Autodesk Inventor part; units mm, degrees
ref_plane "YZ Plane" through (0, 0, 0) normal (1, 0, 0) x (0, 1, 0)
ref_plane "XZ Plane" through (0, 0, 0) normal (0, 1, 0) x (-1, 0, 0)
ref_plane "XY Plane" through (0, 0, 0) normal (0, 0, 1) x (1, 0, 0)
sketch "Sketch1" plane through (0, 0, 0) normal (0, 1, 0) x (-1, 0, 0)
  circle A0 centre (0, 0) radius 40
  dimension "d0" = 80
extrude "Extrusion1" add sketch "Sketch1" along normal blind 6
sketch "Sketch2" plane through (0, 0, 0) normal (0, -1, 0) x (1, 0, 0)
  circle A0 centre (0, 0) radius 35.15
  circle A1 centre (0, 0) radius 24.85
  point P0 (0, 0)
extrude "Extrusion2" cut sketch "Sketch2" against normal blind 1.43
sketch "Sketch3" plane through (0, 6, 0) normal (0, 1, 0) x (1, 0, 0)
  circle A0 centre (-7, 0) radius 0.7835
  circle A1 centre (0, 7) radius 0.7835
  circle A2 centre (0, -7) radius 0.7835
  circle A3 centre (7, 0) radius 0.7835
  point P0 (0, 0)
hole "Hole1" at (-7, 6, 0) at (0, 6, 7) at (7, 6, 0) at (0, 6, -7) direction (0, -1, 0) diameter 2.1 end through all
sketch "Sketch4" plane through (0, 6, 0) normal (0, 1, 0) x (1, 0, 0)
  circle A0 centre (0, 7) radius 1.05
  circle A1 centre (7, 0) radius 1.05
  circle A2 centre (0, -7) radius 1.05
  circle A3 centre (-7, 0) radius 1.05
  circle A4 centre (0, 0) radius 40
  circle A5 centre (-7, 0) radius 2.05
  circle A6 centre (0, -7) radius 2.05
  circle A7 centre (7, 0) radius 2.05
  circle A8 centre (0, 7) radius 2.05
  dimension "d12" = 4.1
extrude "Extrusion3" cut sketch "Sketch4" against normal blind 3 contours A5 | A6 | A7 | A8
sketch "Sketch5" plane through (0, 6, 0) normal (0, 1, 0) x (1, 0, 0)
  circle A0 centre (0, 0) radius 1.75
  circle A1 centre (0, 0) radius 2
  dimension "d27" = 4
extrude "Extrusion4" cut sketch "Sketch5" against normal through all contours A0 | A1
sketch "Sketch6" plane through (0, 0, 0) normal (0, -1, 0) x (1, 0, 0)
  circle A0 centre (0, 0) radius 3
  dimension "d17" = 6
extrude "Extrusion5" cut sketch "Sketch6" against normal blind 1.5
sketch "Sketch7" plane through (0, 6, 0) normal (0, 1, 0) x (1, 0, 0)
  circle A0 centre (-4, -36.56) radius 1.05
  circle A1 centre (-4, -27.06) radius 1.05
  circle A2 centre (14, -27.06) radius 1.05
  circle A3 centre (14, -34.56) radius 1.05
  circle A4 centre (18, 25.06) radius 1.05
  circle A5 centre (18, 32.06) radius 1.05
  circle A6 centre (0, 35.06) radius 1.05
  circle A7 centre (0, 25.06) radius 1.05
  circle A8 centre (-18, 32.06) radius 1.05
  circle A9 centre (-18, 25.06) radius 1.05
  point P0 (0, 0)
hole "Hole2" at (-18, 6, -32.06) at (0, 6, -35.06) at (18, 6, -32.06) at (18, 6, -25.06) at (0, 6, -25.06) at (-18, 6, -25.06) at (-4, 6, 27.06) at (14, 6, 27.06) at (14, 6, 34.56) at (-4, 6, 36.56) direction (0, -1, 0) diameter 1.567 depth 3
properties part number "axis_2_bottom_frame" material "Aluminum 6061-AHC"
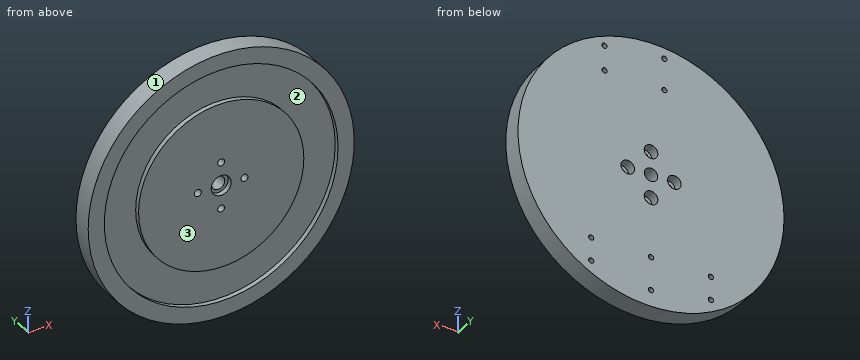
Design review of the part built by this model. Coordinates are the model's own, in mm. Face numbers are marked on the shaded views. Coordinates: 2 decimals unless noted, no trailing zeros. Loops run counter-clockwise (first coordinate to the right, second up) from the corner with the lowest first, then second, coordinate; pieces in that order, holes last.
Q1. For pin 1 (3.5 mm diameter, centred on x = 0, z = 0, fed in from +Y); pin 2 (2 mm diameter, centred on x = 12, y = 5, fed in from -Z); pin 3 (3 mm diameter, centred on x = -0.5, y = 1.5, fed in from -Z); pin 4 (2.5 mm diameter, centred on x = 0, z = 7, fed in from +Y), all flat-tipped, find the tip position at first contact; note any pin that passes through.
Reported:
pin 1: passes through
pin 2: stops at z = -38.46
pin 3: stops at z = -40
pin 4: stops at y = 3
Q2. We need section C-C on x = -15. State the section outline as (y, z) points, and give its area (3 significant figures).
Reported:
outline: (0, -37.08) - (6, -37.08) - (6, 37.08) - (0, 37.08) - (0, 31.79) - (1.43, 31.79) - (1.43, 19.81) - (0, 19.81) - (0, -19.81) - (1.43, -19.81) - (1.43, -31.79) - (0, -31.79) - close
area: 411 mm2
Q3. To check wall thickness, follow line 1 (Z direction, x = 0, y = 4.2); line 2 (Z direction, x = 0, y = 0.65); line 3 (Z direction, x = 16, y = 0.65). State the ranges of each line that lie inside material, in increasing order.
Reported:
line 1: z = -40 to -35.84, -34.28 to -25.84, -24.28 to -9.05, -4.95 to -2, 2 to 4.95, 9.05 to 40
line 2: z = -40 to -35.15, -24.85 to -8.05, -5.95 to -3, 3 to 5.95, 8.05 to 24.85, 35.15 to 40
line 3: z = -36.66 to -31.3, -19.01 to 19.01, 31.3 to 36.66
Q4. We need section D-D on z = -15. State the section outline as (x, y) points.
Reported:
outline: (-37.08, 0) - (-31.79, 0) - (-31.79, 1.43) - (-19.81, 1.43) - (-19.81, 0) - (19.81, 0) - (19.81, 1.43) - (31.79, 1.43) - (31.79, 0) - (37.08, 0) - (37.08, 6) - (-37.08, 6) - close
Q5. The part is to be moulded in two halves that separate along X. For the marked faces 1, 2 and 3, say which applies: +X half, -X half, draft (parallel to the pull), parting line (faces both ways), or undercut.
Reported:
face 1: parting line
face 2: undercut
face 3: draft
Q6. We need section A-A on y = 4.5. State how many separate pieces and enclosed holes the cut face has, and give its area (3 significant figures).
Reported:
separate pieces: 1
enclosed holes: 15
area: 4,940 mm2
